Geometry check sheet. Reference: the model listing, model coordinates, mm. Face numbers are marked on the shaded views. A direction names the side the tool comes from. Round coordinates to 2 decimals unless told otherwise and drop trailing zeros. Loops run counter-clockwise (first coordinate to the right, second up) from the corner with the lowest first, then second, coordinate; pieces in that order, holes last. Notation, with made-up numbers: (44, 29) -> (57, 29) arc R14 cw to (57, 34) -> close; hole circle Ø5 at (-27.75, -0.5). An arc over 180 degrees is marked (long way). Use a Markdown table: item, result. Add a question column.
Q1. Sectioned sample at D-D, the plane y = 7.5. Enter the section's corners in (x, z), then the cut area to 3 significant figures.
Q2. Sectioned sample at A-A, the plane y = 0. Enter the section's corners in (x, z), then the cut area to 3 significant figures.
Q3. Release check for a two-part mould opening along X. For the marked faces 1, 2 and 3 record: released by +X, released by -X, zero draft, split by the parting line, or undercut.
Q4. Material ranges on L1, parallel to Y at x = 13, z = 3.5; L2, parallel to X at y = 14.5, z = 2; L3, parallel to X at y = 5, z = 7, recorded low to high.
Q5. Gauge pin test, flat ends, axial feed: P1, Ø1, axis at x = -10.5, z = -2, coming from the +Y side; P2, Ø6, axis at x = 2, z = -3, coming from the -Y side (3 decimals); P3, Ø4, axis at x = -6.5, z = 1.5, coming from the -Y side. Record the tip position at first contact, or that the pin passes through.
Q6. Sectioned sample at C-C, the plane x = -8. Enter the section's corners in (y, z).
Q7. Set-up check for the marked faces 4 and 5: record each of +Z, -Z, +X, -X, +Y, -Y from which the full face is reachable in a straight line by a thin tool's end or side.
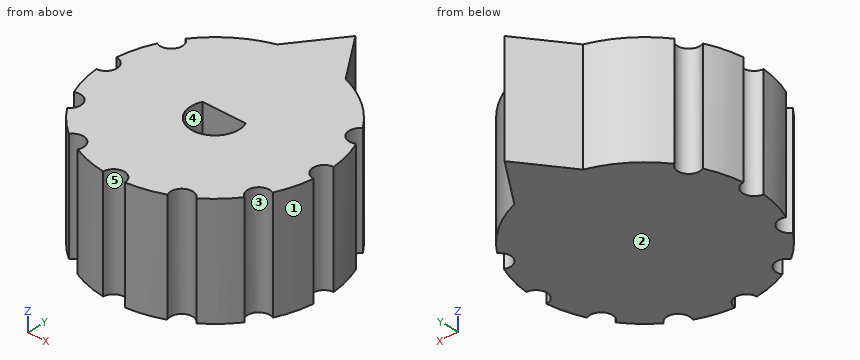
```python
from build123d import *

# Parameters (mm, degrees)
F0_R     = 15
F1_DEPTH = 10
F2_R     = 15
F3_DEPTH = 5
F5_DEPTH = 15
F6_DEPTH = 15


# Not quite as in the source:
# - a feature names something its author has since deleted; it is built from what else it names


with BuildPart() as f1:
    # F0 (on Top) → F1 (new body)
    with BuildSketch(Plane.XY):
        Circle(F0_R)
        with BuildLine():
            ThreePointArc((2.9510768453, 1.3614864865), (0, -3.25), (-2.9510768453, 1.3614864865))
            Line((-2.9510768453, 1.3614864865), (2.9510768453, 1.3614864865))
        make_face(mode=Mode.SUBTRACT)
    extrude(amount=F1_DEPTH)

    # F2 (on face) → F3 (join)
    with BuildSketch(Plane(origin=(0, 0, 0), x_dir=(1, 0, 0), z_dir=(0, 0, -1))):
        Circle(F2_R)
        with BuildLine():
            ThreePointArc((-2.9510768453, -1.3614864865), (0, 3.25), (2.9510768453, -1.3614864865))
            Line((2.9510768453, -1.3614864865), (-2.9510768453, -1.3614864865))
        make_face(mode=Mode.SUBTRACT)
        with BuildLine():
            Line((-2.9510768453, -1.3614864865), (2.9510768453, -1.3614864865))
            ThreePointArc((2.9510768453, -1.3614864865), (0, 3.25), (-2.9510768453, -1.3614864865))
        make_face()
    extrude(amount=F3_DEPTH)

    # F4 (on face) → F5 (join)
    with BuildSketch(Plane.XY.offset(10)):
        with BuildLine():
            Line((4.707880128, 14.2420456642), (0, 20.7567233592))
            Line((0, 20.7567233592), (-4.707880128, 14.2420456642))
            ThreePointArc((-4.707880128, 14.2420456642), (0, 15), (4.707880128, 14.2420456642))
        make_face()
    extrude(amount=-F5_DEPTH)

    # F4 (on face) → F6 (cut, through all)
    with BuildSketch(Plane.XY.offset(10)):
        with BuildLine():
            ThreePointArc((13.6744910648, 6.1650867081), (12.9903810568, 7.5), (12.1763672382, 8.7599132919))
            ThreePointArc((12.1763672382, 8.7599132919), (11.6913429511, 6.75), (13.6744910648, 6.1650867081))
        make_face()
        with BuildLine():
            ThreePointArc((15, 0), (14.9812382666, 0.75), (14.925, 1.4981238267))
            ThreePointArc((14.925, 1.4981238267), (13.5, 0), (14.925, -1.4981238267))
            ThreePointArc((14.925, -1.4981238267), (14.9812382666, -0.75), (15, 0))
        make_face()
        with BuildLine():
            ThreePointArc((12.1763672382, -8.7599132919), (12.9903810568, -7.5), (13.6744910648, -6.1650867081))
            ThreePointArc((13.6744910648, -6.1650867081), (11.6913429511, -6.75), (12.1763672382, -8.7599132919))
        make_face()
        with BuildLine():
            ThreePointArc((6.1650867081, -13.6744910648), (7.5, -12.9903810568), (8.7599132919, -12.1763672382))
            ThreePointArc((8.7599132919, -12.1763672382), (6.75, -11.6913429511), (6.1650867081, -13.6744910648))
        make_face()
        with BuildLine():
            ThreePointArc((1.4981238267, -14.925), (0, -13.5), (-1.4981238267, -14.925))
            ThreePointArc((-1.4981238267, -14.925), (0, -15), (1.4981238267, -14.925))
        make_face()
        with BuildLine():
            ThreePointArc((-6.1650867081, -13.6744910648), (-6.75, -11.6913429511), (-8.7599132919, -12.1763672382))
            ThreePointArc((-8.7599132919, -12.1763672382), (-7.5, -12.9903810568), (-6.1650867081, -13.6744910648))
        make_face()
        with BuildLine():
            ThreePointArc((-12.1763672382, -8.7599132919), (-11.6913429511, -6.75), (-13.6744910648, -6.1650867081))
            ThreePointArc((-13.6744910648, -6.1650867081), (-12.9903810568, -7.5), (-12.1763672382, -8.7599132919))
        make_face()
        with BuildLine():
            ThreePointArc((-14.925, -1.4981238267), (-13.5, 0), (-14.925, 1.4981238267))
            ThreePointArc((-14.925, 1.4981238267), (-15, 0), (-14.925, -1.4981238267))
        make_face()
        with BuildLine():
            ThreePointArc((-13.6744910648, 6.1650867081), (-11.6913429511, 6.75), (-12.1763672382, 8.7599132919))
            ThreePointArc((-12.1763672382, 8.7599132919), (-12.9903810568, 7.5), (-13.6744910648, 6.1650867081))
        make_face()
    extrude(amount=-F6_DEPTH, mode=Mode.SUBTRACT)


solid = f1.part
```
Values:
| question | item | result |
|---|---|---|
| 1 | outline | (-11.49, -5) -> (11.49, -5) -> (11.49, 10) -> (-11.49, 10) -> close |
| 1 | area | 345 mm^2 |
| 2 | outline | (-13.5, -5) -> (13.5, -5) -> (13.5, 10) -> (3.25, 10) -> (3.25, 0) -> (-3.25, 0) -> (-3.25, 10) -> (-13.5, 10) -> close |
| 2 | area | 340 mm^2 |
| 3 | face 1 | released by +X |
| 3 | face 2 | zero draft |
| 3 | face 3 | undercut |
| 4 | L1 | -6 to 6 |
| 4 | L2 | -4.52 to 4.52 |
| 4 | L3 | -14.14 to 14.14 |
| 5 | P1 | y = 11.18 |
| 5 | P2 | y = -14.925 |
| 5 | P3 | y = -14.31 |
| 6 | outline | (-11.58, -5) -> (12.69, -5) -> (12.69, 10) -> (-11.58, 10) -> close |
| 7 | face 4 | +Z |
| 7 | face 5 | +Z, -Z, -Y |
